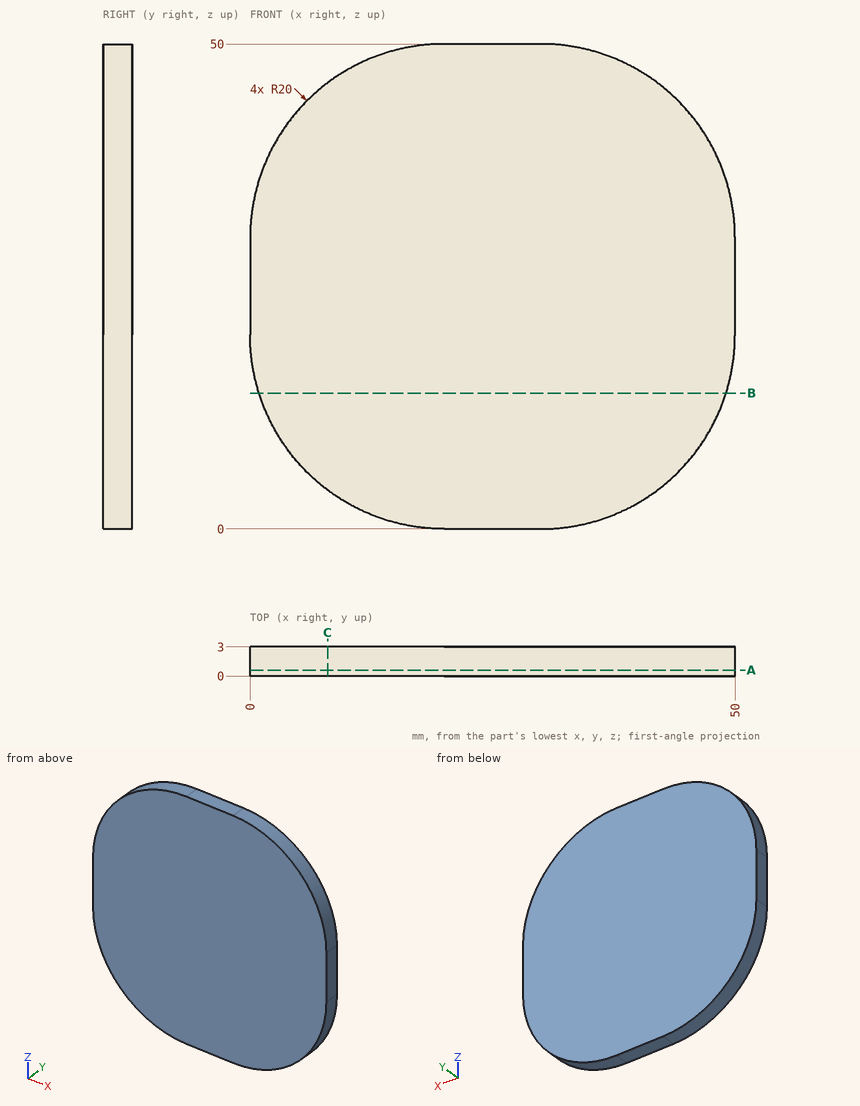
Design review of the part shown in the three views and the two pictorial views. Dimensions are in mm from the part's minimum x, y and z. Round coordinates to 2 decimals unless told otherwise and drop trailing zeros. Write each loop counter-clockwise with the first axis right and the second up, starting at its lowest first coordinate (ties: lowest second). Pieces come first, ordered by that corner, then holes. Notation, with made-up numbers: (-29, 20.25) -> (-1, 20.25) arc R21 cw to (-1, 51.25) -> close; hole circle Ø9 at (76, 2.25). An arc over 180 degrees is marked (long way). Answer as a JSON object with one key per item and string values.
1. We need section C-C on x = 8. State the section outline as (y, z) points.
Results found:
{"outline": "(0, 4) -> (3, 4) -> (3, 46) -> (0, 46) -> close"}
2. Clearance check with a flat-ended pin moving along its axis: pin 1 (1 mm diameter, centred on x = 31, y = 0.5, fed in from -Z). State where the tip first meets the part, or that it passes through.
Results found:
{"pin 1": "stops at z = 0.01"}
3. We need section B-B on z = 14. State the section outline as (x, y) points.
Results found:
{"outline": "(0.92, 0) -> (49.08, 0) -> (49.08, 3) -> (0.92, 3) -> close"}
4. To check wall thickness, follow line 1 along X through (y, z) = (2.45, 15.5); line 2 along Z through (x, y) = (33, 1.8); line 3 along Z through (x, y) = (31, 0.75). State the ranges of each line that lie inside material, in increasing order.
Results found:
{"line 1": "x = 0.51 to 49.49", "line 2": "z = 0.23 to 49.77", "line 3": "z = 0.03 to 49.97"}
5. We need section A-A on y = 0.6. State the section outline as (x, z) points.
Results found:
{"outline": "(0, 20) arc R20 ccw to (20, 0) -> (30, 0) arc R20 ccw to (50, 20) -> (50, 30) arc R20 ccw to (30, 50) -> (20, 50) arc R20 ccw to (0, 30) -> close"}
